from build123d import *

# Parameters (mm, degrees)
BOSS_EXTRU_1_DEPTH           = 200
ENL_V_MAT_EXTRU_1_DEPTH      = 100
ESQUISSE3_W                  = 300
ESQUISSE3_H                  = 210
BOSS_EXTRU_2_DEPTH           = 3
ENL_V_MAT_EXTRU_2_DEPTH      = 299.654946406
ENL_V_MAT_EXTRU_2_DEPTH_BACK = 299.654946406
ESQUISSE4_R                  = 5.25


with BuildPart() as part:
    # Esquisse1 → Boss.-Extru.1 (new body)
    with BuildSketch(Plane(origin=(0, 0, 0), x_dir=(1, 0, 0), z_dir=(0, 1, 0))):
        with BuildLine():
            Line((-12, -15), (12, -15))
            ThreePointArc((12, -15), (14.121320344, -14.121320344), (15, -12))
            Line((15, -12), (15, 12))
            ThreePointArc((15, 12), (14.121320344, 14.121320344), (12, 15))
            Line((12, 15), (-12, 15))
            ThreePointArc((-12, 15), (-14.121320344, 14.121320344), (-15, 12))
            Line((-15, 12), (-15, -12))
            ThreePointArc((-15, -12), (-14.121320344, -14.121320344), (-12, -15))
        make_face()
        with BuildLine():
            Line((-10, -13), (10, -13))
            ThreePointArc((10, -13), (12.121320344, -12.121320344), (13, -10))
            Line((13, -10), (13, 10))
            ThreePointArc((13, 10), (12.121320344, 12.121320344), (10, 13))
            Line((10, 13), (-10, 13))
            ThreePointArc((-10, 13), (-12.121320344, 12.121320344), (-13, 10))
            Line((-13, 10), (-13, -10))
            ThreePointArc((-13, -10), (-12.121320344, -12.121320344), (-10, -13))
        make_face(mode=Mode.SUBTRACT)
    extrude(amount=BOSS_EXTRU_1_DEPTH)

    # Esquisse2 → Enlèv. mat.-Extru.1 (cut)
    with BuildSketch(Plane(origin=(15, 0, 0), x_dir=(0, 0, -1), z_dir=(1, 0, 0))):
        Polygon((15, 200), (-15, 140), (-15, 200), align=None)
    extrude(amount=-ENL_V_MAT_EXTRU_1_DEPTH, mode=Mode.SUBTRACT)

    # Esquisse3 → Boss.-Extru.2 (add)
    with BuildSketch(Plane(origin=(0, 34, 68), x_dir=(1, 0, 0), z_dir=(0, 0.447213595499958, 0.8944271909999159))):
        with Locations((0, 152.05262247)):
            Rectangle(ESQUISSE3_W, ESQUISSE3_H)
    extrude(amount=BOSS_EXTRU_2_DEPTH)

    # Esquisse4 → Enlèv. mat.-Extru.2 (cut, two sides: drawn at the far end of the back side and taken through both)
    with BuildSketch(Plane(origin=(0, 34, 68), x_dir=(1, 0, 0), z_dir=(0, 0.447213595499958, 0.8944271909999159)).offset(-ENL_V_MAT_EXTRU_2_DEPTH_BACK)):
        with Locations(Location((-110, 217.05262247, 0), (0, 0, 90))):
            Circle(ESQUISSE4_R)
        with Locations(Location((110, 217.05262247, 0), (0, 0, 90))):
            Circle(ESQUISSE4_R)
        with Locations(Location((110, 87.05262247, 0), (0, 0, 90))):
            Circle(ESQUISSE4_R)
        with Locations(Location((-110, 87.05262247, 0), (0, 0, 90))):
            Circle(ESQUISSE4_R)
    extrude(amount=ENL_V_MAT_EXTRU_2_DEPTH + ENL_V_MAT_EXTRU_2_DEPTH_BACK, mode=Mode.SUBTRACT)


solid = part.part
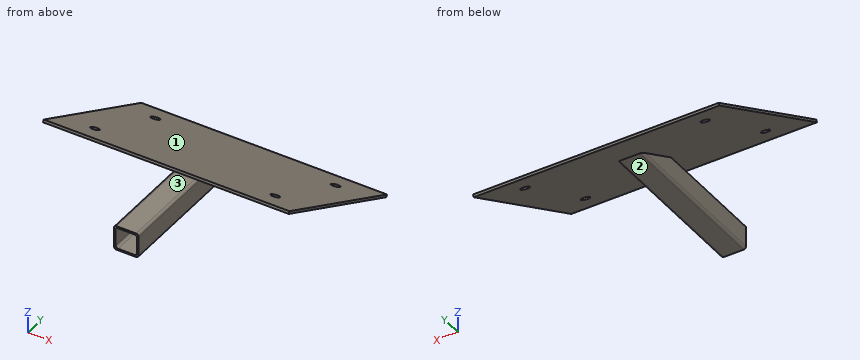
Could you check a few things on this model? Use its own coordinates, in mm. Face numbers are marked on the shaded views. Give positions to 0.01 mm unless a question says otherwise; leave off trailing zeros. Order: outer loops, then holes, each group sorted by start corner. A loop starts at its lowest first (then second) coordinate and runs counter-clockwise, first axis right, second up.
Item 1: If we mould it in two halves opening along Z, with no side actions, what happens to the marked faces 1, 2 and 3? For each: pulls with the +Z half, pulls with the -Z half, needs draft (parallel to the pull), parting line crosses it, or undercut.
Item 2: I need wall thicknesses on line 1 (X direction, y = 52.5, z = 8.5); line 2 (Z direction, x = 1, y = 127); line 3 (Z direction, x = 6.5, y = 167). Which ranges of each line are inside material? Lowest first, please.
Item 3: I'm going to push flat-ended pins straight in: pin 1 (3 mm diameter, centred on x = 100.5, z = 17.5, fed in from -Y); pin 2 (10 mm diameter, centred on x = 4, y = 83, fed in from +Z); pin 3 (19 mm diameter, centred on x = -1, y = 142, fed in from -Z); pin 4 (8 mm diameter, centred on y = 177, z = -20, fed in from -X). Where does each tip first touch, or does it pass through?
Item 4: If we section it at B-B, the plane y = 96.5: Write out the boundary of the cut face in (x, z), plus the area to 3 significant figures.
Item 5: If we section it at A-A, the plane y = 53.5: Write out the boundary of the cut face in (x, z).
Item 6: If we section it at C-C, the plane z = 1: Write out the boundary of the cut face in (x, y).
Item 7: If we section it at D-D, the plane x = -91.5: Write out the boundary of the cut face in (y, z).
Values:
1. face 1: pulls with the +Z half
1. face 2: pulls with the -Z half
1. face 3: undercut
2. line 1: x = -15 to -13, 13 to 15
2. line 2: z = -15 to -13, 13 to 15, 21.5 to 24.85
2. line 3: z = -15 to -13, 1.5 to 4.85
3. pin 1: stops at y = 132
3. pin 2: stops at z = 49.35
3. pin 3: stops at z = -15
3. pin 4: passes through
4. outline: (-150, 36.75) - (150, 36.75) - (150, 40.1) - (-150, 40.1) - close; (-15, -12) arc R3 ccw to (-12, -15) - (12, -15) arc R3 ccw to (15, -12) - (15, 12) arc R3 ccw to (12, 15) - (-12, 15) arc R3 ccw to (-15, 12) - close; hole (-13, -10) arc R3 ccw to (-10, -13) - (10, -13) arc R3 ccw to (13, -10) - (13, 10) arc R3 ccw to (10, 13) - (-10, 13) arc R3 ccw to (-13, 10) - close
4. area: 1,230 mm2
5. outline: (-15, -12) arc R3 ccw to (-12, -15) - (12, -15) arc R3 ccw to (15, -12) - (15, 12) arc R3 ccw to (12, 15) - (-12, 15) arc R3 ccw to (-15, 12) - close; hole (-13, -10) arc R3 ccw to (-10, -13) - (10, -13) arc R3 ccw to (13, -10) - (13, 10) arc R3 ccw to (10, 13) - (-10, 13) arc R3 ccw to (-13, 10) - close
6. outline: (-150, 168) - (-15, 168) - (-15, 0) - (-13, 0) - (-13, 168) - (13, 168) - (13, 0) - (15, 0) - (15, 168) - (150, 168) - (150, 174.71) - (-150, 174.71) - close
7. outline: (76.09, 46.96) - (263.91, -46.96) - (265.26, -44.27) - (77.43, 49.64) - close
